```python
from build123d import *

# Parameters (mm, degrees)
F1_DEPTH = 48
F2_R     = 2.65
F3_DEPTH = 5
F4_R     = 19
F4_R_2   = 1.7
F5_DEPTH = 5
F6_ANGLE = 40
F7_ANGLE = 90
F8_R     = 2


with BuildPart() as f1:
    # F0 (on Top) → F1 (new body)
    with BuildSketch(Plane.XY):
        Polygon((-1.8198511713, 5), (-20, 5), (-20, 0), (0, 0), (38.1642201468, 32.0235830494), (34.9502820984, 35.853805265), align=None)
    extrude(amount=F1_DEPTH)

    # F2 (on face) → F3 (cut, through all)
    with BuildSketch(Plane(origin=(0, 5, 0), x_dir=(-1, 0, 0), z_dir=(0, 1, 0))):
        with Locations((10, 10)):
            Circle(F2_R)
        with Locations((10, 38)):
            Circle(F2_R)
    extrude(amount=-F3_DEPTH, mode=Mode.SUBTRACT)

    # F4 (on face) → F5 (cut, through all)
    with BuildSketch(Plane(origin=(-3.2139380484, 3.8302222156, 0), x_dir=(-0.7660444431, -0.6427876097, 0), z_dir=(-0.6427876097, 0.7660444431, 0))):
        with Locations((-25.8198511713, 24)):
            Circle(F4_R)
        with Locations((-9.8198511713, 40)):
            Circle(F4_R_2)
        with Locations((-9.8198511713, 8)):
            Circle(F4_R_2)
        with Locations((-41.8198511713, 8)):
            Circle(F4_R_2)
        with Locations((-41.8198511713, 40)):
            Circle(F4_R_2)
    extrude(amount=-F5_DEPTH, mode=Mode.SUBTRACT)


with BuildPart() as f1_1:
    # F6: moved
    add(f1.part.rotate(Axis((0, 0, 24), (0, 0, -1)), F6_ANGLE))


with BuildPart() as f1_2:
    # F7: moved
    add(f1_1.part.rotate(Axis((24.9099255857, 0, 0), (1, 0, 0)), F7_ANGLE))

    # F8
    f8_edges = [f1_2.edges().sort_by_distance(p)[0] for p in [
        (1.819851, -24, 5),
        (0, -24, 0),
        (-13.71392, 0, 14.770863),
        (-13.71392, -48, 14.770863),
        (49.819851, 0, 2.5),
        (49.819851, -48, 2.5),
    ]]
    fillet(f8_edges, radius=F8_R)


solid = f1_2.part
```
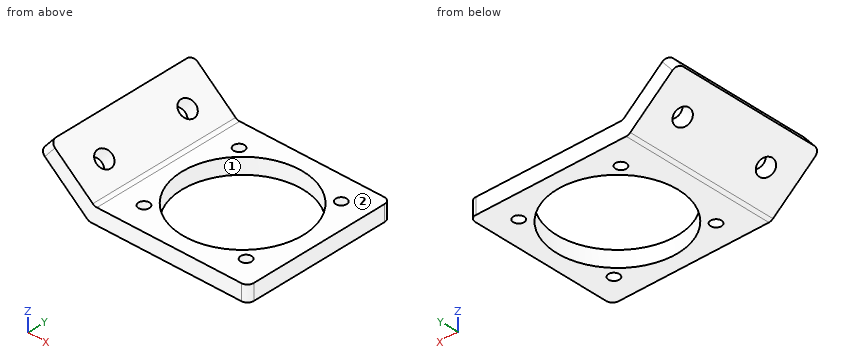
Check sheet for the modelled part. Datum: model origin and axes. Units: mm. Face numbers are marked on the shaded views. Give positions to 0.01 mm unless a question says otherwise; leave off trailing zeros. Write each loop counter-clockwise with the first axis right and the second up, starting at its lowest first coordinate (ties: lowest second). Pieces come first, ordered by that corner, then holes. Notation, with made-up numbers: (-35, 30.25) - (-7, 30.25) arc R9 cw to (-7, 37.25) - close; hole circle Ø6 at (77, 0.25). An arc over 180 degrees is marked (long way). Answer as a JSON object with one key per item and string values. Group by question number.
1) Sectioned sample at B-B (x = 20). Record the cut outline in (y, z), then the cut area to 3 significant figures.
2) Sectioned sample at C-C (x = 27.5). Record the cut outline in (y, z), then the cut area to 3 significant figures.
3) Depth check by flat-ended pin: P1, Ø5.5, axis at x = 9.82, y = -8, coming from the -Z side; P2, Ø1.5, axis at y = -36, z = 5.5, coming from the -X side (3 decimals); P3, Ø4, axis at x = 43, y = -12.5, coming from the +Z side; P4, Ø4, axis at y = -34.5, z = 6.5, coming from the -X side. Enter the tip coordinate at first touch or a pass-through.
4) Sectioned sample at A-A (y = -24). Record the cut outline in (x, z).
5) Thickness scan on probe 1 along X at (y, z) = (-8, 1.7); probe 2 along X at (y, z) = (-8, 3); probe 3 along Z at (x, y) = (25, -3). Record the ranges inside material, lowest first. Write a range as from..to.
6) Release check for a two-part mould opening along Y. For the marked faces 1 and 2 record: pulls with the +Y half, pulls with the -Y half, needs draft (parallel to the pull), parting line crosses it, or undercut.
Geometry results:
{
 "1": {"outline": "(-48, 0) - (-42.09, 0) - (-42.09, 5) - (-48, 5) - close; (-5.91, 0) - (0, 0) - (0, 5) - (-5.91, 5) - close", "area": "59.1 mm^2"},
 "2": {"outline": "(-48, 0) - (-42.93, 0) - (-42.93, 5) - (-48, 5) - close; (-5.07, 0) - (0, 0) - (0, 5) - (-5.07, 5) - close", "area": "50.7 mm^2"},
 "3": {"P1": "stops at z = 0", "P2": "stops at x = -7.145", "P3": "stops at z = 5", "P4": "stops at x = -10.13"},
 "4": {"outline": "(-15.32, 12.86) - (-0.56, 0.47) arc R2 ccw to (0.73, 0) - (6.82, 0) - (6.82, 5) - (2.55, 5) arc R2 cw to (1.26, 5.47) - (-12.11, 16.69) - close; (44.82, 0) - (49.82, 0) - (49.82, 5) - (44.82, 5) - close"},
 "5": {"probe 1": "x = -2.03..8.12, 11.52..15.57, 36.07..40.12, 43.52..49.82", "probe 2": "x = -3.58..8.12, 11.52..15.57, 36.07..40.12, 43.52..49.82", "probe 3": "z = 0..5"},
 "6": {"face 1": "undercut", "face 2": "needs draft"}
}
